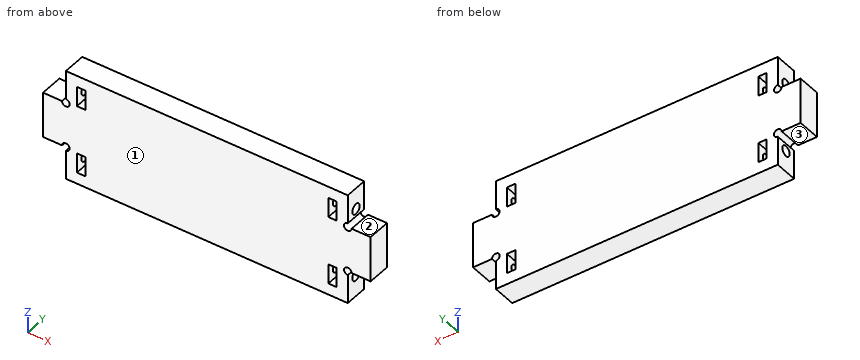
Autodesk Inventor part; units mm, degrees
ref_plane "우측면도" through (0, 0, 0) normal (1, 0, 0) x (0, 1, 0)
ref_plane "평면도" through (0, 0, 0) normal (0, 1, 0) x (-1, 0, 0)
ref_plane "정면도" through (0, 0, 0) normal (0, 0, 1) x (1, 0, 0)
sketch "스케치1" plane through (0, 0, 0) normal (0, 1, 0) x (-1, 0, 0)
  line L0 (-37, 14.6) -> (37, 14.6)
  line L1 (37, 14.6) -> (37, -14.6)
  line L2 (37, -14.6) -> (-37, -14.6)
  line L3 (-37, -14.6) -> (-37, 14.6)
  line L4 (-37, 14.6) -> (37, -14.6) construction
  line L5 (37, 14.6) -> (-37, -14.6) construction
  line L6 (37, 6) -> (43, 6)
  line L7 (43, 6) -> (43, -6)
  line L8 (43, -6) -> (37, -6)
  line L9 (37, -6) -> (37, 6)
  line L10 (-37, 6) -> (-43, 6)
  line L11 (-43, 6) -> (-43, -6)
  line L12 (-43, -6) -> (-37, -6)
  line L13 (-37, -6) -> (-37, 6)
  point P0 (0, 0)
  dimension "d0" = 74
  dimension "d1" = 29.2
  dimension "d2" = 6
  dimension "d3" = 12
  dimension "d4" = 6
  dimension "d5" = 12
extrude "돌출1" add sketch "스케치1" along normal blind 6
sketch "스케치2" plane through (43, 0, 6) normal (1, 0, 0) x (0, 0, -1)
  line L0 (12, 0) -> (20.6, 0)
  line L1 (20.6, 0) -> (20.6, 6)
  line L2 (12, 6) -> (20.6, 6)
  line L3 (12, 0) -> (12, 6)
  line L4 (-8.6, 0) -> (0, 0)
  line L5 (0, 0) -> (0, 6)
  line L6 (-8.6, 6) -> (0, 6)
  line L7 (-8.6, 0) -> (-8.6, 6)
  circle A0 centre (15, 3) radius 1.35
  circle A1 centre (-3, 3) radius 1.35
  point P0 (6, 0)
  dimension "d8" = 2.7
  dimension "d9" = 2.7
extrude "돌출2" cut sketch "스케치2" against normal blind 14 contours A0 | A1
sketch "스케치3" plane through (-43, 0, -6) normal (-1, 0, 0) x (0, 0, 1)
  line L0 (12, 0) -> (20.6, 0)
  line L1 (20.6, 0) -> (20.6, 6)
  line L2 (12, 6) -> (20.6, 6)
  line L3 (12, 0) -> (12, 6)
  circle A0 centre (-3, 3) radius 1.35
  line L4 (-8.6, 0) -> (0, 0)
  line L5 (0, 0) -> (0, 6)
  line L6 (-8.6, 6) -> (0, 6)
  line L7 (-8.6, 0) -> (-8.6, 6)
  circle A1 centre (15, 3) radius 1.35
  circle A2 centre (-3, 3) radius 1.35
  circle A3 centre (15, 3) radius 1.35
  point P0 (6, 0)
extrude "돌출3" cut sketch "스케치3" against normal blind 14 contours A0 | A1
sketch "스케치4" plane through (0, 6, 0) normal (0, 1, 0) x (1, 0, 0)
  line L0 (37, -14.6) -> (37, -6)
  line L1 (37, -6) -> (43, -6)
  line L2 (43, -6) -> (43, 6)
  line L3 (43, 6) -> (37, 6)
  line L4 (37, 6) -> (37, 14.6)
  line L5 (37, 14.6) -> (-37, 14.6)
  line L6 (-37, 14.6) -> (-37, 6)
  line L7 (-37, 6) -> (-43, 6)
  line L8 (-43, 6) -> (-43, -6)
  line L9 (-43, -6) -> (-37, -6)
  line L10 (-37, -6) -> (-37, -14.6)
  line L11 (-37, -14.6) -> (37, -14.6)
  line L12 (-37, 10.35) -> (-29, 10.35)
  line L13 (-37, 7.65) -> (-29, 7.65)
  line L14 (-33, 10.35) -> (-33, 7.65)
  line L15 (-34.1, 6.4) -> (-31.9, 6.4)
  line L16 (-31.9, 6.4) -> (-31.9, 11.6)
  line L17 (-31.9, 11.6) -> (-34.1, 11.6)
  line L18 (-34.1, 11.6) -> (-34.1, 6.4)
  line L19 (-34.1, 6.4) -> (-31.9, 11.6) construction
  line L20 (-31.9, 6.4) -> (-34.1, 11.6) construction
  line L21 (34.1, 6.4) -> (31.9, 6.4)
  line L22 (31.9, 6.4) -> (31.9, 11.6)
  line L23 (31.9, 11.6) -> (34.1, 11.6)
  line L24 (34.1, 11.6) -> (34.1, 6.4)
  line L25 (34.1, 6.4) -> (31.9, 11.6) construction
  line L26 (31.9, 6.4) -> (34.1, 11.6) construction
  line L27 (31.9, -11.6) -> (34.1, -11.6)
  line L28 (34.1, -11.6) -> (34.1, -6.4)
  line L29 (34.1, -6.4) -> (31.9, -6.4)
  line L30 (31.9, -6.4) -> (31.9, -11.6)
  line L31 (31.9, -11.6) -> (34.1, -6.4) construction
  line L32 (34.1, -11.6) -> (31.9, -6.4) construction
  line L33 (-34.1, -11.6) -> (-31.9, -11.6)
  line L34 (-31.9, -11.6) -> (-31.9, -6.4)
  line L35 (-31.9, -6.4) -> (-34.1, -6.4)
  line L36 (-34.1, -6.4) -> (-34.1, -11.6)
  line L37 (-34.1, -11.6) -> (-31.9, -6.4) construction
  line L38 (-31.9, -11.6) -> (-34.1, -6.4) construction
  point P0 (0, 0)
  point P1 (-33, 9)
  point P2 (33, 9)
  point P3 (33, -9)
  point P4 (-33, -9)
  dimension "d14" = 2.2
  dimension "d15" = 5.2
  dimension "d16" = 2.2
  dimension "d17" = 5.2
  dimension "d18" = 2.2
  dimension "d19" = 5.2
  dimension "d20" = 2.2
  dimension "d21" = 5.2
extrude "돌출4" cut sketch "스케치4" against normal blind 14 contours L18 L12 L14 L13 | L13 L16 L15 L18 | L18 L17 L16 L12 | L14 L12 L16 L13 | L21 L22 L23 L24 | L30 L29 L28 L27 | L36 L35 L34 L33
sketch "스케치5" plane through (0, 6, 0) normal (0, 1, 0) x (1, 0, 0)
  line L0 (31.9, 6.4) -> (31.9, 11.6)
  line L1 (31.9, 11.6) -> (34.1, 11.6)
  line L2 (34.1, 11.6) -> (34.1, 6.4)
  line L3 (34.1, 6.4) -> (31.9, 6.4)
  line L4 (-34.1, -6.4) -> (-31.9, -6.4)
  line L5 (-31.9, -6.4) -> (-31.9, -11.6)
  line L6 (-31.9, -11.6) -> (-34.1, -11.6)
  line L7 (-34.1, -11.6) -> (-34.1, -6.4)
  line L8 (31.9, -6.4) -> (34.1, -6.4)
  line L9 (34.1, -6.4) -> (34.1, -11.6)
  line L10 (34.1, -11.6) -> (31.9, -11.6)
  line L11 (31.9, -11.6) -> (31.9, -6.4)
  line L12 (-34.1, 6.4) -> (-34.1, 11.6)
  line L13 (-34.1, 11.6) -> (-31.9, 11.6)
  line L14 (-31.9, 11.6) -> (-31.9, 6.4)
  line L15 (-31.9, 6.4) -> (-34.1, 6.4)
  line L16 (37, -14.6) -> (37, -6)
  line L17 (37, -6) -> (43, -6)
  line L18 (43, -6) -> (43, 6)
  line L19 (43, 6) -> (37, 6)
  line L20 (37, 6) -> (37, 14.6)
  line L21 (37, 14.6) -> (-37, 14.6)
  line L22 (-37, 14.6) -> (-37, 6)
  line L23 (-37, 6) -> (-43, 6)
  line L24 (-43, 6) -> (-43, -6)
  line L25 (-43, -6) -> (-37, -6)
  line L26 (-37, -6) -> (-37, -14.6)
  line L27 (-37, -14.6) -> (37, -14.6)
  circle A0 centre (-37, -6) radius 1
  circle A1 centre (-37, 6) radius 1
  circle A2 centre (37, -6) radius 1
  circle A3 centre (37, 6) radius 1
  point P0 (0, 0)
  point P1 (-37, -7)
  point P2 (-38, -6)
  dimension "d24" = 2
  dimension "d25" = 2
  dimension "d26" = 2
  dimension "d27" = 2
extrude "돌출5" cut sketch "스케치5" against normal through all contours A2 L17 L16 | L16 L17 A2 | L26 L25 A0 | A3 L20 L19 | L19 L20 A3 | A1 L22 L23 | L23 L22 A1 picked at (-37.657, -5.9202)
properties part number "body front connection" material "PMMA 플라스틱"
CAD build for the part. Positions are in the model's coordinates, mm. Face numbers are marked on the shaded views. A direction names the side the tool comes from. Round coordinates to 2 decimals unless told otherwise and drop trailing zeros. Loops run counter-clockwise (first coordinate to the right, second up) from the corner with the lowest first, then second, coordinate; pieces in that order, holes last. Notation, with made-up numbers: M -7,69.25 L 32,69.25 A8 cw 32,74.25 Z; hole C -3,-23 d7. An arc over 180 degrees is marked long. Use a Markdown table: item, result. Add a question column.
(1) Cut at A-A (z = 9). Give the cut face in (x, y).
(2) Which spindle directions (+Z, -Z, +X, -X, +Y, -Y) get a long thin tool onto all of the face, cutting with end or side? Do the marked faces 1, 2 and 3. Say none if no direction does.
(3) Drill centre lines: line 1 (X direction, y = 1.65, z = -7.5); line 2 (Z direction, x = 33.5, y = 2.5); line 3 (Y direction, x = -30.6, z = -9). Where is each one in solid material? Low to high.
(4) Cut at C-C (z = -8.75). Give the cut face in (x, y).
(5) Flat gauge pin, fed straight in: pin 1 (2.5 mm diameter, centred on y = 3, z = 9, fed in from +X). Where does the tip first touch, or does it go through?
(6) Cut at B-B (y = 0.8). State how many separate pieces and enclosed holes the cut face has, and give its area (3 significant figures).
Geometry says:
| question | item | result |
|---|---|---|
| 1 | outline | M -37,0 L -34.1,0 L -34.1,1.65 L -37,1.65 Z; M -37,4.35 L -34.1,4.35 L -34.1,6 L -37,6 Z; M -31.9,0 L 31.9,0 L 31.9,1.65 L 29,1.65 L 29,4.35 L 31.9,4.35 L 31.9,6 L -31.9,6 L -31.9,4.35 L -29,4.35 L -29,1.65 L -31.9,1.65 Z; M 34.1,0 L 37,0 L 37,1.65 L 34.1,1.65 Z; M 34.1,4.35 L 37,4.35 L 37,6 L 34.1,6 Z |
| 2 | face 1 | +Z, -Z, +X, -X, -Y |
| 2 | face 2 | +Z, +X, +Y, -Y |
| 2 | face 3 | -Z, -X, +Y, -Y |
| 3 | line 1 | x = -37 to -34.1, -31.9 to 31.9, 34.1 to 37 |
| 3 | line 2 | z = -14.6 to -11.6, -6.4 to 6.4, 11.6 to 14.6 |
| 3 | line 3 | y = 0 to 1.65, 4.35 to 6 |
| 4 | outline | M -37,0 L -34.1,0 L -34.1,1.67 L -37,1.67 Z; M -37,4.33 L -34.1,4.33 L -34.1,6 L -37,6 Z; M -31.9,0 L 31.9,0 L 31.9,1.67 L 29,1.67 L 29,4.33 L 31.9,4.33 L 31.9,6 L -31.9,6 L -31.9,4.33 L -29,4.33 L -29,1.67 L -31.9,1.67 Z; M 34.1,0 L 37,0 L 37,1.67 L 34.1,1.67 Z; M 34.1,4.33 L 37,4.33 L 37,6 L 34.1,6 Z |
| 5 | pin 1 | stops at x = 29 |
| 6 | separate pieces | 1 |
| 6 | enclosed holes | 4 |
| 6 | area | 2,250 mm² |
